For this review, take the finished solid that the model builds, in its own axes (mm). A direction names the side the tool comes from. Coordinates: 2 decimals unless noted, no trailing zeros. Loops run counter-clockwise (first coordinate to the right, second up) from the corner with the lowest first, then second, coordinate; pieces in that order, holes last. Notation, with made-up numbers: (16, -26.75) - (39, -26.75) arc R21 cw to (39, -18.75) - close; hole circle Ø9 at (82.5, 66). An arc over 180 degrees is marked (long way). Answer as a JSON object with one key per item and string values. Group by question number.
Item 1: Tool access review of faces 3 (the flat face through (-145, 5, 2)), 4 (the flat face through (-75.313, -24, 8)), 5 (the flat face through (-37, -5, 2)): name each direction out of +Z, -Z, +X, -X, +Y, -Y from which nothing blocks a thin tool from reaching the whole face with its end or side.
Item 2: Clearance check with flat-ended pins moving along their axes: pin 1 (3 mm diameter, centred on x = -162, z = 8, fed in from +Y); pin 2 (5.5 mm diameter, centred on x = -14, z = 3.5, fed in from -Y); pin 3 (1.5 mm diameter, centred on x = -109, z = 3, fed in from -Y); pin 4 (4 mm diameter, centred on x = -32, z = 5.5, fed in from +Y). State where each tip first meets the part, or that it passes through.
Item 3: We need section A-A (z = 9.25). Give the boundary of the cut face in (x, y).
Item 4: To check wall thickness, follow line 1 (Y direction, x = -47, z = 6.25); line 2 (Y direction, x = -90, z = 8.75); line 3 (X direction, y = -10.5, z = 8.75). State the ranges of each line that lie inside material, in increasing order.
Item 5: We need section B-B (y = -17). Give the boundary of the cut face in (x, z).
Item 6: We need section C-C (x = -166). Give the boundary of the cut face in (y, z), then the cut area to 3 significant figures.
Item 7: Mouldability with a two-part tool opening along X and no side actions: class faces 1 (the flat face through (-53, -19, 12)), 2 (the cylindrical face through (-165, 10, 2)) as released by +X, released by -X, zero draft, split by the parting line, or undercut.
from build123d import *
from build123d import SkipClean  # not in build123d's __all__

# Parameters (mm, degrees)
F1_DEPTH = 5
F3_DEPTH = 7


with BuildPart() as f1:
    # F0 (on Top) → F1 (new body)
    with BuildSketch(Plane.XY):
        with BuildLine():
            ThreePointArc((0, 5), (3.5355339059, 3.5355339059), (5, 0))
            ThreePointArc((5, 0), (3.5355339059, -3.5355339059), (0, -5))
            Line((0, -5), (-8.6602540378, -5))
            ThreePointArc((-8.6602540378, -5), (2.588190451, -9.6592582629), (10, 0))
            ThreePointArc((10, 0), (2.588190451, 9.6592582629), (-8.6602540378, 5))
            Line((-8.6602540378, 5), (0, 5))
        make_face()
        with BuildLine():
            ThreePointArc((0, -5), (-5, 0), (0, 5))
            Line((0, 5), (-8.6602540378, 5))
            ThreePointArc((-8.6602540378, 5), (-10, 0), (-8.6602540378, -5))
            Line((-8.6602540378, -5), (0, -5))
        make_face()
        with BuildLine():
            ThreePointArc((-8.6602540378, -5), (-10, 0), (-8.6602540378, 5))
            Line((-8.6602540378, 5), (-16.3397459622, 5))
            ThreePointArc((-16.3397459622, 5), (-15.3407417371, 2.588190451), (-15, 0))
            ThreePointArc((-15, 0), (-15.3407417371, -2.588190451), (-16.3397459622, -5))
            Line((-16.3397459622, -5), (-8.6602540378, -5))
        make_face()
        with BuildLine():
            ThreePointArc((-15, 0), (-15.3407417371, 2.588190451), (-16.3397459622, 5))
            Line((-16.3397459622, 5), (-33.6602540378, 5))
            ThreePointArc((-33.6602540378, 5), (-35, 0), (-33.6602540378, -5))
            Line((-33.6602540378, -5), (-16.3397459622, -5))
            ThreePointArc((-16.3397459622, -5), (-15.3407417371, -2.588190451), (-15, 0))
        make_face()
        with BuildLine():
            Line((-33.6602540378, 5), (-16.3397459622, 5))
            ThreePointArc((-16.3397459622, 5), (-25, 10), (-33.6602540378, 5))
        make_face()
        with BuildLine():
            ThreePointArc((-33.6602540378, -5), (-25, -10), (-16.3397459622, -5))
            Line((-16.3397459622, -5), (-33.6602540378, -5))
        make_face()
        with BuildLine():
            ThreePointArc((-33.6602540378, -5), (-35, 0), (-33.6602540378, 5))
            Line((-33.6602540378, 5), (-40.4196010845, 5))
            ThreePointArc((-40.4196010845, 5), (-40.1050843164, 2.5087878084), (-40, 0))
            ThreePointArc((-40, 0), (-40.1050843164, -2.5087878084), (-40.4196010845, -5))
            Line((-40.4196010845, -5), (-33.6602540378, -5))
        make_face()
        with BuildLine():
            ThreePointArc((-40, 0), (-40.1050843164, 2.5087878084), (-40.4196010845, 5))
            Line((-40.4196010845, 5), (-50.635083269, 5))
            ThreePointArc((-50.635083269, 5), (-50.1594060747, 2.5200858497), (-50, 0))
            ThreePointArc((-50, 0), (-50.1594060747, -2.5200858497), (-50.635083269, -5))
            Line((-50.635083269, -5), (-40.4196010845, -5))
            ThreePointArc((-40.4196010845, -5), (-40.1050843164, -2.5087878084), (-40, 0))
        make_face()
        with BuildLine():
            Line((-50.635083269, 5), (-40.4196010845, 5))
            ThreePointArc((-40.4196010845, 5), (-70, 30), (-99.5803989155, 5))
            Line((-99.5803989155, 5), (-89.364916731, 5))
            ThreePointArc((-89.364916731, 5), (-70, 20), (-50.635083269, 5))
        make_face()
        with BuildLine():
            ThreePointArc((-99.5803989155, -5), (-70, -30), (-40.4196010845, -5))
            Line((-40.4196010845, -5), (-50.635083269, -5))
            ThreePointArc((-50.635083269, -5), (-70, -20), (-89.364916731, -5))
            Line((-89.364916731, -5), (-99.5803989155, -5))
        make_face()
        with BuildLine():
            ThreePointArc((-99.5803989155, -5), (-100, 0), (-99.5803989155, 5))
            Line((-99.5803989155, 5), (-116.3397459622, 5))
            ThreePointArc((-116.3397459622, 5), (-115.3407417371, 2.588190451), (-115, 0))
            ThreePointArc((-115, 0), (-115.3407417371, -2.588190451), (-116.3397459622, -5))
            Line((-116.3397459622, -5), (-99.5803989155, -5))
        make_face()
        with BuildLine():
            Line((-89.364916731, 5), (-99.5803989155, 5))
            ThreePointArc((-99.5803989155, 5), (-100, 0), (-99.5803989155, -5))
            Line((-99.5803989155, -5), (-89.364916731, -5))
            ThreePointArc((-89.364916731, -5), (-90, 0), (-89.364916731, 5))
        make_face()
        with BuildLine():
            ThreePointArc((-115, 0), (-115.3407417371, 2.588190451), (-116.3397459622, 5))
            Line((-116.3397459622, 5), (-133.6602540378, 5))
            ThreePointArc((-133.6602540378, 5), (-135, 0), (-133.6602540378, -5))
            Line((-133.6602540378, -5), (-116.3397459622, -5))
            ThreePointArc((-116.3397459622, -5), (-115.3407417371, -2.588190451), (-115, 0))
        make_face()
        with BuildLine():
            Line((-133.6602540378, 5), (-116.3397459622, 5))
            ThreePointArc((-116.3397459622, 5), (-125, 10), (-133.6602540378, 5))
        make_face()
        with BuildLine():
            ThreePointArc((-133.6602540378, -5), (-125, -10), (-116.3397459622, -5))
            Line((-116.3397459622, -5), (-133.6602540378, -5))
        make_face()
        with BuildLine():
            ThreePointArc((-133.6602540378, -5), (-135, 0), (-133.6602540378, 5))
            Line((-133.6602540378, 5), (-156.3397459622, 5))
            ThreePointArc((-156.3397459622, 5), (-155.3407417371, 2.588190451), (-155, 0))
            ThreePointArc((-155, 0), (-155.3407417371, -2.588190451), (-156.3397459622, -5))
            Line((-156.3397459622, -5), (-133.6602540378, -5))
        make_face()
        with BuildLine():
            ThreePointArc((-155, 0), (-155.3407417371, 2.588190451), (-156.3397459622, 5))
            Line((-156.3397459622, 5), (-173.6602540378, 5))
            ThreePointArc((-173.6602540378, 5), (-175, 0), (-173.6602540378, -5))
            Line((-173.6602540378, -5), (-156.3397459622, -5))
            ThreePointArc((-156.3397459622, -5), (-155.3407417371, -2.588190451), (-155, 0))
        make_face()
        with BuildLine():
            Line((-173.6602540378, 5), (-156.3397459622, 5))
            ThreePointArc((-156.3397459622, 5), (-165, 10), (-173.6602540378, 5))
        make_face()
        with BuildLine():
            ThreePointArc((-173.6602540378, -5), (-165, -10), (-156.3397459622, -5))
            Line((-156.3397459622, -5), (-173.6602540378, -5))
        make_face()
        with BuildLine():
            ThreePointArc((-173.6602540378, -5), (-175, 0), (-173.6602540378, 5))
            Line((-173.6602540378, 5), (-191.3397459622, 5))
            ThreePointArc((-191.3397459622, 5), (-190.3407417371, 2.588190451), (-190, 0))
            ThreePointArc((-190, 0), (-190.3407417371, -2.588190451), (-191.3397459622, -5))
            Line((-191.3397459622, -5), (-173.6602540378, -5))
        make_face()
        with BuildLine():
            ThreePointArc((-190, 0), (-190.3407417371, 2.588190451), (-191.3397459622, 5))
            Line((-191.3397459622, 5), (-200, 5))
            ThreePointArc((-200, 5), (-196.4644660941, 3.5355339059), (-195, 0))
            ThreePointArc((-195, 0), (-196.4644660941, -3.5355339059), (-200, -5))
            Line((-200, -5), (-191.3397459622, -5))
            ThreePointArc((-191.3397459622, -5), (-190.3407417371, -2.588190451), (-190, 0))
        make_face()
        with BuildLine():
            Line((-200, 5), (-191.3397459622, 5))
            ThreePointArc((-191.3397459622, 5), (-210, 0), (-191.3397459622, -5))
            Line((-191.3397459622, -5), (-200, -5))
            ThreePointArc((-200, -5), (-205, 0), (-200, 5))
        make_face()
    extrude(amount=F1_DEPTH)

    # F2 (on face) → F3 (join)
    with BuildSketch(Plane.XY.offset(5)):
        with BuildLine():
            ThreePointArc((-75.3128379583, -19.2814354452), (-84.2561475764, -14.0271970215), (-89.364916731, -5))
            Line((-89.364916731, -5), (-99.5803989155, -5))
            ThreePointArc((-99.5803989155, -5), (-91.3251821922, -21.1006304282), (-75.3128379583, -29.5258150239))
            Line((-75.3128379583, -29.5258150239), (-75.3128379583, -19.2814354452))
        make_face()
        with BuildLine():
            ThreePointArc((-41.0863354104, 8), (-71.5365980819, 29.9606219284), (-99.5803989155, 5))
            Line((-99.5803989155, 5), (-89.364916731, 5))
            ThreePointArc((-89.364916731, 5), (-71.5866967281, 19.9369604878), (-51.6696972202, 8))
            Line((-51.6696972202, 8), (-41.0863354104, 8))
        make_face()
        with BuildLine():
            ThreePointArc((-64.9254471064, -29.5677005012), (-49.8731234875, -22.2465467399), (-41.0863354104, -8))
            Line((-41.0863354104, -8), (-51.6696972202, -8))
            ThreePointArc((-51.6696972202, -8), (-56.9951167094, -15.1945059346), (-64.9254471064, -19.345514026))
            Line((-64.9254471064, -19.345514026), (-64.9254471064, -29.5677005012))
        make_face()
    with SkipClean():  # cleaning this boolean's faces spoils the solid; the shape is the same uncleaned
        extrude(amount=F3_DEPTH)


solid = f1.part
Check sheet entries:
{
 "1": {"face 3": "+Z, -Z, +Y", "face 4": "+Z, -Y", "face 5": "+Z, -Z, -Y"},
 "2": {"pin 1": "passes through", "pin 2": "stops at y = -5.65", "pin 3": "stops at y = -5", "pin 4": "stops at y = 8.62"},
 "3": {"outline": "(-99.58, -5) arc R30 ccw to (-75.31, -29.53) - (-75.31, -19.28) arc R20 cw to (-89.36, -5) - close; (-99.58, 5) - (-89.36, 5) arc R20 cw to (-51.67, 8) - (-41.09, 8) arc R30 ccw to start; (-64.93, -29.57) arc R30 ccw to (-41.09, -8) - (-51.67, -8) arc R20 cw to (-64.93, -19.35) - close"},
 "4": {"line 1": "y = -19.26 to -8, 8 to 19.26", "line 2": "y = -22.36 to -5, 5 to 22.36", "line 3": "x = -98.1 to -87.02, -52.98 to -41.9"},
 "5": {"outline": "(-94.72, 0) - (-80.54, 0) - (-80.54, 12) - (-94.72, 12) - close; (-59.46, 0) - (-45.28, 0) - (-45.28, 12) - (-59.46, 12) - close"},
 "6": {"outline": "(-9.95, 0) - (9.95, 0) - (9.95, 5) - (-9.95, 5) - close", "area": "99.5 mm2"},
 "7": {"face 1": "zero draft", "face 2": "undercut"}
}
